from build123d import *

# Parameters (mm, degrees)
SKETCH4_R           = 2.5
BOSS_EXTRUDE2_DEPTH = 32
BOSS_EXTRUDE3_DEPTH = 28.5
SKETCH1_W           = 12
SKETCH1_H           = 23
BOSS_EXTRUDE4_DEPTH = 22
BOSS_EXTRUDE6_DEPTH = 2
FILLET2_R           = 0.5


with BuildPart() as part:
    # Sketch4 → Boss-Extrude2 (new body)
    with BuildSketch(Plane(origin=(0, 0, 0), x_dir=(1, 0, 0), z_dir=(0, 1, 0))):
        with Locations((51.314367453, -99.151596437)):
            Circle(SKETCH4_R)
    extrude(amount=BOSS_EXTRUDE2_DEPTH)

    # Sketch3 → Boss-Extrude3 (add)
    with BuildSketch(Plane(origin=(0, 0, 0), x_dir=(1, 0, 0), z_dir=(0, 1, 0))):
        with BuildLine():
            Line((48.814367453, -106.151596437), (48.814367453, -104.605952495))
            ThreePointArc((48.814367453, -104.605952495), (51.314367453, -93.151596437), (53.814367453, -104.605952495))
            Line((53.814367453, -104.605952495), (53.814367453, -106.151596437))
            ThreePointArc((53.814367453, -106.151596437), (51.314367453, -108.651596437), (48.814367453, -106.151596437))
        make_face()
    extrude(amount=BOSS_EXTRUDE3_DEPTH)

    # Sketch1 → Boss-Extrude4 (add)
    with BuildSketch(Plane(origin=(0, 0, 0), x_dir=(1, 0, 0), z_dir=(0, 1, 0))):
        with Locations((51.314367453, -104.651596437)):
            Rectangle(SKETCH1_W, SKETCH1_H)
    extrude(amount=BOSS_EXTRUDE4_DEPTH)

    # Sketch7 → Boss-Extrude6 (add)
    with BuildSketch(Plane(origin=(0, 16, 0), x_dir=(1, 0, 0), z_dir=(0, 1, 0))):
        with BuildLine():
            Line((52.694479243, -120.651596437), (57.314367453, -120.651596437))
            Line((57.314367453, -120.651596437), (57.314367453, -116.151596437))
            Line((57.314367453, -116.151596437), (45.314367453, -116.151596437))
            Line((45.314367453, -116.151596437), (45.314367453, -120.651596437))
            Line((45.314367453, -120.651596437), (49.994479243, -120.651596437))
            ThreePointArc((49.994479243, -120.651596437), (51.344479243, -116.601596437), (52.694479243, -120.651596437))
        make_face()
        with BuildLine():
            Line((45.314367453, -93.151596437), (57.314367453, -93.151596437))
            Line((57.314367453, -93.151596437), (57.314367453, -88.651596437))
            Line((57.314367453, -88.651596437), (52.694479243, -88.651596437))
            ThreePointArc((52.694479243, -88.651596437), (51.344479243, -92.701596437), (49.994479243, -88.651596437))
            Line((49.994479243, -88.651596437), (45.314367453, -88.651596437))
            Line((45.314367453, -88.651596437), (45.314367453, -93.151596437))
        make_face()
    extrude(amount=BOSS_EXTRUDE6_DEPTH)

    # Fillet2
    fillet2_edges = [part.edges().sort_by_distance(p)[0] for p in [
        (45.314367453, 17, 120.651596437),
        (57.314367453, 17, 120.651596437),
        (45.314367453, 17, 88.651596437),
        (57.314367453, 17, 88.651596437),
    ]]
    fillet(fillet2_edges, radius=FILLET2_R)


solid = part.part
For this review, take the finished solid that the model builds, in its own axes (mm). A direction names the side the tool comes from. Give positions to 0.01 mm unless a question says otherwise; leave off trailing zeros. Loops run counter-clockwise (first coordinate to the right, second up) from the corner with the lowest first, then second, coordinate; pieces in that order, holes last. Notation, with made-up numbers: M 74,-37 L 130,-37 A17 ccw 130,-23 Z; hole C 46.25,77.5 d8. An arc over 180 degrees is marked long. Answer as a JSON object with one key per item and string values. Group by question number.
Q1. Tool access review of faces 1 (the flat face through (51, 18, 93)), 2 (the flat face through (51.2, 18, 116.4)), 3 (the flat face through (46.5, 22, 94.6)), 4 (the cylindrical face through (53.7, 30.2, 98.4)), 5 (the flat face through (51, 8, 93.152)): name each direction out of +Z, -Z, +X, -X, +Y, -Y from which nothing blocks a thin tool from reaching the whole face with its end or side.
Q2. Add section C-C on y = 26.5. Give the boundary of the cut face in (x, z).
Q3. For probe 1 along Z at (x, y) = (50.75, 5.5); probe 2 along Y at (x, z) = (56.75, 115.5); probe 3 along Z at (x, y) = (53, 16.5), list the stretches that pass through material, from the lowest coordinate up. Write a range as [from, to].
Q4. Add section D-D on x = 55.75. Give the boundary of the cut face in (y, z).
Q5. Add section B-B on x = 49.5. Give the boundary of the cut face in (y, z), and give its area (3 significant figures).
Q6. Insertion check: P1, Ø2, axis at x = 51.5, z = 91, coming from the +Y side; P2, Ø1.7, axis at y = 26, z = 105.5, coming from the +X side; P3, Ø3.5, axis at x = 51.5, y = 6.5, coming from the +Z side; P4, Ø6, axis at x = 49, z = 108.5, coming from the +Y side. Each pin has a flat end and moves straight along its axis. Give the tip position at first contact, or say it passes through.
Q7. Add section A-A on z = 117.5. Give the boundary of the cut face in (x, y), and give its area (3 significant figures).
Checked values:
{
 "1": {"face 1": "-Z, +X, -X, +Y", "face 2": "+Z, +X, -X, +Y", "face 3": "-Z, -X, +Y", "face 4": "+Y", "face 5": "-Z, +X, -X, -Y"},
 "2": {"outline": "M 48.81,104.61 A6 ccw long 53.81,104.61 L 53.81,106.15 A2.5 ccw 48.81,106.15 Z"},
 "3": {"probe 1": "[93.15, 116.15]", "probe 2": "[0, 22]", "probe 3": "[88.65, 88.93], [91.98, 117.33], [120.38, 120.65]"},
 "4": {"outline": "M 0,93.15 L 16,93.15 L 16,88.65 L 18,88.65 L 18,93.15 L 22,93.15 L 22,95.11 L 28.5,95.11 L 28.5,103.19 L 22,103.19 L 22,116.15 L 18,116.15 L 18,120.65 L 16,120.65 L 16,116.15 L 0,116.15 Z"},
 "5": {"outline": "M 0,93.15 L 16,93.15 L 16,91.74 L 18,91.74 L 18,93.15 L 22,93.15 L 22,93.43 L 28.5,93.43 L 28.5,97.43 L 32,97.43 L 32,100.87 L 28.5,100.87 L 28.5,107.87 L 22,107.87 L 22,116.15 L 18,116.15 L 18,117.56 L 16,117.56 L 16,116.15 L 0,116.15 Z; M 16,88.65 L 18,88.65 L 18,89.16 L 16,89.16 Z; M 16,120.14 L 18,120.14 L 18,120.65 L 16,120.65 Z", "area": "620 mm²"},
 "6": {"P1": "through", "P2": "x = 53.81", "P3": "z = 116.15", "P4": "y = 28.5"},
 "7": {"outline": "M 45.31,16 L 49.55,16 L 49.55,18 L 45.31,18 Z; M 53.14,16 L 57.31,16 L 57.31,18 L 53.14,18 Z", "area": "16.8 mm²"}
}
